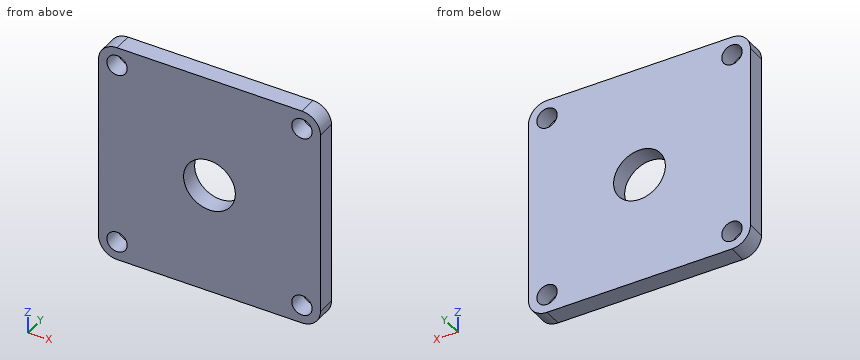
from build123d import *

# Parameters (mm, degrees)
SKETCH1_W           = 60
SKETCH1_H           = 60
BOSS_EXTRUDE1_DEPTH = 5
SKETCH2_R           = 2.75
CUT_EXTRUDE1_DEPTH  = 5
FILLET2_R           = 5
SKETCH3_R           = 7
CUT_EXTRUDE2_DEPTH  = 5


with BuildPart() as part:
    # Sketch1 → Boss-Extrude1 (new body)
    with BuildSketch(Plane(origin=(0, 0, 0), x_dir=(1, 0, 0), z_dir=(0, 1, 0))):
        Rectangle(SKETCH1_W, SKETCH1_H)
    extrude(amount=BOSS_EXTRUDE1_DEPTH)

    # Sketch2 → Cut-Extrude1 (cut)
    with BuildSketch(Plane(origin=(0, 5, 0), x_dir=(1, 0, 0), z_dir=(0, 1, 0))):
        with Locations((25, 25)):
            Circle(SKETCH2_R)
        with Locations((-25, 25)):
            Circle(SKETCH2_R)
        with Locations((-25, -25)):
            Circle(SKETCH2_R)
        with Locations((25, -25)):
            Circle(SKETCH2_R)
    extrude(amount=-CUT_EXTRUDE1_DEPTH, mode=Mode.SUBTRACT)

    # Fillet2
    fillet2_edges = [part.edges().sort_by_distance(p)[0] for p in [
        (-30, 2.5, -30),
        (30, 2.5, -30),
        (30, 2.5, 30),
        (-30, 2.5, 30),
    ]]
    fillet(fillet2_edges, radius=FILLET2_R)

    # Sketch3 → Cut-Extrude2 (cut)
    with BuildSketch(Plane(origin=(0, 5, 0), x_dir=(1, 0, 0), z_dir=(0, 1, 0))):
        Circle(SKETCH3_R)
    extrude(amount=-CUT_EXTRUDE2_DEPTH, mode=Mode.SUBTRACT)


solid = part.part
Here's how the part is built. I have some questions about the finished solid (model axes, mm). Coordinates: 2 decimals unless noted, no trailing zeros. Order: outer loops, then holes, each group sorted by start corner. A loop starts at its lowest first (then second) coordinate and runs counter-clockwise, first axis right, second up. Notation, with made-up numbers: M 32.5,-0.5 L 41.5,-0.5 A15 cw 41.5,17.5 Z; hole C 50,9 d2. An arc over 180 degrees is marked long. Answer as CSV lines item,"result". Start each with the question number.
1. I want a section at D-D, the plane x = -26. Write out the boundary of the cut face in (y, z).
2. I want a section at C-C, the plane y = 1.05. Write out the boundary of the cut face in (x, z).
3. I want a section at B-B, the plane x = 0. Write out the boundary of the cut face in (y, z), and give its area (3 significant figures).
4. I want a section at A-A, the plane z = 0. Write out the boundary of the cut face in (x, y), and give its area (3 significant figures).
5. I need wall thicknesses on line 1 (Z direction, x = 25, y = 2.4); line 2 (Z direction, x = -27, y = 3.55). Which ranges of each line are inside material? Lowest first, please. Write a range as [from, to].
Recorded:
1,outline,"M 0,-29.9 L 5,-29.9 L 5,-27.56 L 0,-27.56 Z; M 0,-22.44 L 5,-22.44 L 5,22.44 L 0,22.44 Z; M 0,27.56 L 5,27.56 L 5,29.9 L 0,29.9 Z"
2,outline,"M -30,-25 A5 ccw -25,-30 L 25,-30 A5 ccw 30,-25 L 30,25 A5 ccw 25,30 L -25,30 A5 ccw -30,25 Z; hole C -25,-25 d5.5; hole C -25,25 d5.5; hole C 0,0 d14; hole C 25,-25 d5.5; hole C 25,25 d5.5"
3,outline,"M 0,-30 L 5,-30 L 5,-7 L 0,-7 Z; M 0,7 L 5,7 L 5,30 L 0,30 Z"
3,area,"230 mm2"
4,outline,"M -30,0 L -7,0 L -7,5 L -30,5 Z; M 7,0 L 30,0 L 30,5 L 7,5 Z"
4,area,"230 mm2"
5,line 1,"z = [-30, -27.75], [-22.25, 22.25], [27.75, 30]"
5,line 2,"z = [-29.58, -26.89], [-23.11, 23.11], [26.89, 29.58]"
